from build123d import *

# Parameters (mm, degrees)
SKETCH_1_W          = 86
SKETCH_1_H          = 25
EXTRUDE_1_DEPTH     = 7
SKETCH_2_W          = 15
SKETCH_2_H          = 17
CUT_EXTRUDE_1_DEPTH = 90.833178726
SKETCH_3_W          = 55
SKETCH_3_H          = 13
CUT_EXTRUDE_2_DEPTH = 5.2
SKETCH_4_W          = 55
SKETCH_4_H          = 7.5
CUT_EXTRUDE_3_DEPTH = 2
SKETCH_5_R          = 1.8
CUT_EXTRUDE_4_DEPTH = 90.699498326
SKETCH_6_R          = 1.4
CUT_EXTRUDE_5_DEPTH = 90.699498326
CUT_EXTRUDE_6_DEPTH = 90.710868907
CHAMFER_1_SIZE      = 1
SKETCH_8_W          = 82
SKETCH_8_H          = 48
EXTRUDE_2_DEPTH     = 2.8


with BuildPart() as part:
    # 草图1 → 凸台-拉伸1 (new body)
    with BuildSketch(Plane.XY):
        with Locations((43, 12.5)):
            Rectangle(SKETCH_1_W, SKETCH_1_H)
    extrude(amount=EXTRUDE_1_DEPTH)

    # 草图2 → 切除-拉伸1 (cut, through all)
    with BuildSketch(Plane.XY.offset(7)):
        with Locations((77.5, 14.5)):
            Rectangle(SKETCH_2_W, SKETCH_2_H)
    extrude(amount=-CUT_EXTRUDE_1_DEPTH, mode=Mode.SUBTRACT)

    # 草图3 → 切除-拉伸2 (cut)
    with BuildSketch(Plane.XY.offset(7)):
        with Locations((42.5, 16.5)):
            Rectangle(SKETCH_3_W, SKETCH_3_H)
    extrude(amount=-CUT_EXTRUDE_2_DEPTH, mode=Mode.SUBTRACT)

    # 草图4 → 切除-拉伸3 (cut)
    with BuildSketch(Plane.XY.offset(7)):
        with Locations((42.5, 6.25)):
            Rectangle(SKETCH_4_W, SKETCH_4_H)
    extrude(amount=-CUT_EXTRUDE_3_DEPTH, mode=Mode.SUBTRACT)

    # 草图5 → 切除-拉伸4 (cut, through all)
    with BuildSketch(Plane.XY.offset(5)):
        with Locations((64, 7)):
            Circle(SKETCH_5_R)
        with Locations((54.5, 7)):
            Circle(SKETCH_5_R)
        with Locations((23.5, 7)):
            Circle(SKETCH_5_R)
    extrude(amount=-CUT_EXTRUDE_4_DEPTH, mode=Mode.SUBTRACT)

    # 草图6 → 切除-拉伸5 (cut, through all)
    with BuildSketch(Plane.XY.offset(5)):
        with Locations((59, 7)):
            Circle(SKETCH_6_R)
        with Locations((28.5, 7)):
            Circle(SKETCH_6_R)
    extrude(amount=-CUT_EXTRUDE_5_DEPTH, mode=Mode.SUBTRACT)

    # 草图7 → 切除-拉伸6 (cut, through all)
    with BuildSketch(Plane.XY.offset(1.8)):
        with BuildLine():
            Line((23, 19.5), (40, 19.5))
            ThreePointArc((40, 19.5), (43, 16.5), (40, 13.5))
            Line((40, 13.5), (23, 13.5))
            ThreePointArc((23, 13.5), (20, 16.5), (23, 19.5))
        make_face()
        with BuildLine():
            Line((48, 19.5), (65, 19.5))
            ThreePointArc((65, 19.5), (68, 16.5), (65, 13.5))
            Line((65, 13.5), (48, 13.5))
            ThreePointArc((48, 13.5), (45, 16.5), (48, 19.5))
        make_face()
    extrude(amount=-CUT_EXTRUDE_6_DEPTH, mode=Mode.SUBTRACT)

    # 倒角1
    chamfer_1_edges = [part.edges().sort_by_distance(p)[0] for p in [
        (42.5, 10, 5),
    ]]
    chamfer(chamfer_1_edges, length=CHAMFER_1_SIZE)

    # 草图8 → 凸台-拉伸2 (add)
    with BuildSketch(Plane(origin=(0, 0, 0), x_dir=(-1, 0, 0), z_dir=(0, 0, -1))):
        Polygon((-95, 38), (-92, 38), (-92, 44), (-89, 44), (-89, -56), (3, -56), (3, 44), (6, 44), (6, 38), (9, 38), (9, 48), (-2, 48), (-2, 44), (-84, 44), (-84, 48), (-95, 48), align=None)
        Polygon((-86, 0), (0, 0), (0, 25), (-2, 25), (-2, 40), (-84, 40), (-84, 25), (-86, 25), align=None, mode=Mode.SUBTRACT)
        with Locations((-43, -26)):
            Rectangle(SKETCH_8_W, SKETCH_8_H, mode=Mode.SUBTRACT)
    extrude(amount=-EXTRUDE_2_DEPTH)


solid = part.part
Can you work these out from the model? Positions are in its coordinate system, mm. A direction names the side the tool comes from. Round coordinates to 2 decimals unless told otherwise and drop trailing zeros. Write each loop counter-clockwise with the first axis right and the second up, starting at its lowest first coordinate (ties: lowest second). Pieces come first, ordered by that corner, then holes. Notation, with made-up numbers: M 81,-7.75 L 124,-7.75 A5 ccw 124,-3.75 Z; hole C -5.75,46.25 d6. An arc over 180 degrees is marked long. Use a Markdown table: item, result.
Item 1: We'd pull the mould along Y, two halves only. Please class faces 6 (the face through (44, -50, 1)), 7 (the face through (-9, 43, 1)), 8 (the face through (42, 0, 5)): released by +Y, released by -Y, zero draft, split by the parting line, or undercut.
Found:
| item | result |
|---|---|
| face 6 | undercut |
| face 7 | zero draft |
| face 8 | released by -Y |
Item 2: I want a section at A-A (x = 28.5). State how many separate pieces and enclosed holes the cut face has, and give its area (3 significant figures).
Found:
| item | result |
|---|---|
| separate pieces | 5 |
| enclosed holes | 0 |
| area | 101 mm2 |
Item 3: For pin 1 Ø1 at (x, z) = (56, 5) entering from +Y; pin 2 Ø1.5 at (y, z) = (17.5, 3.5) entering from +X; pin 3 Ø2 at (x, z) = (53, 1) entering from +Y, each with a flat end and sliding along its axis, tell me the tip position at first contact or that it passes through.
Found:
| item | result |
|---|---|
| pin 1 | stops at y = 25 |
| pin 2 | stops at x = 89 |
| pin 3 | stops at y = 44 |
Item 4: I want a section at B-B (y = 16.5). List the corners of the cut face in (x, z) for me, and give its area (3 significant figures).
Found:
| item | result |
|---|---|
| outline | M -3,0 L 20,0 L 20,1.8 L 15,1.8 L 15,7 L 0,7 L 0,2.8 L -3,2.8 Z; M 43,0 L 45,0 L 45,1.8 L 43,1.8 Z; M 68,0 L 70,0 L 70,1.8 L 68,1.8 Z; M 85,0 L 89,0 L 89,2.8 L 86,2.8 L 86,7 L 85,7 Z |
| area | 145 mm2 |
Item 5: I want a section at C-C (y = 35.5). List the corners of the cut face in (x, z) for me, and give its area (3 significant figures).
Found:
| item | result |
|---|---|
| outline | M -3,0 L 2,0 L 2,2.8 L -3,2.8 Z; M 84,0 L 89,0 L 89,2.8 L 84,2.8 Z |
| area | 28.0 mm2 |
Item 6: If I drill on line 1 along Y through (x, z) = (4.5, 1.5); line 2 along Y through (x, z) = (27, 1.25); line 3 along Y through (x, z) = (43.5, 2.5), over which ranges is the centre line in solid material (lowest first)? Write a range as [from, to].
Found:
| item | result |
|---|---|
| line 1 | y = [-56, -50], [-2, 25], [40, 44] |
| line 2 | y = [-56, -50], [-2, 13.5], [19.5, 25], [40, 44] |
| line 3 | y = [-56, -50], [-2, 10], [23, 25], [40, 44] |
Item 7: Which directions (+Z, -Z, +X, -X, +Y, -Y) give clear straight access to the entire face, cutting with the end or side of a thin tool? Please do faces 1 (the face through (0, 12, 5)), 2 (the face through (-4, 48, 1)), 3 (the face through (77, 6, 4)), 4 (the face through (50, 23, 4)), 5 (the face through (86, 12, 5)).
Found:
| item | result |
|---|---|
| face 1 | +Z, -X, +Y, -Y |
| face 2 | +Z, -Z, +X, -X, +Y |
| face 3 | +Z, -Z |
| face 4 | +Z |
| face 5 | +Z, +X, +Y, -Y |
